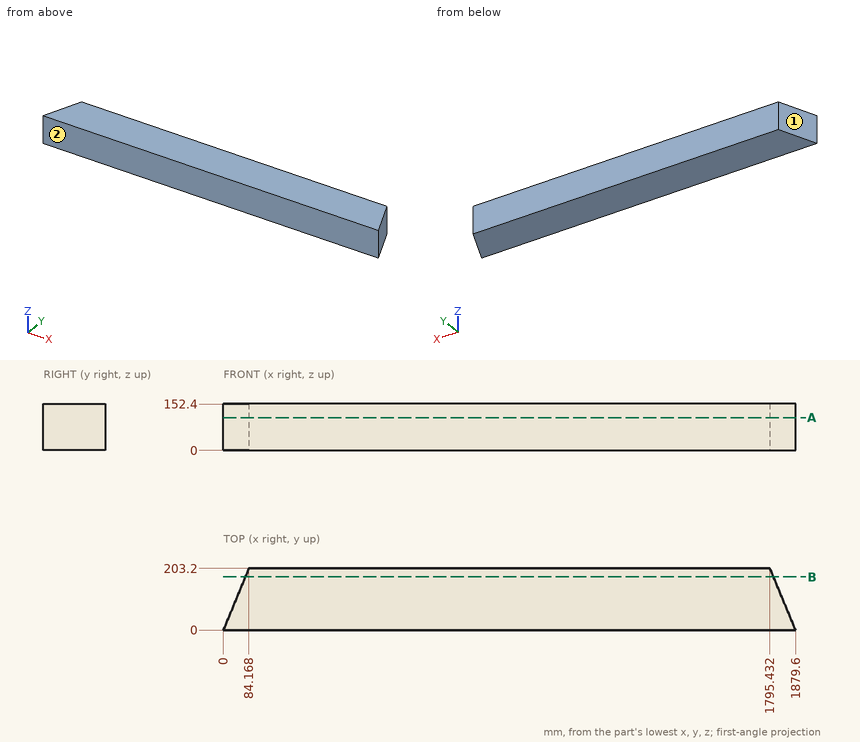
Input: dimensioned drawing with shaded views. Units: mm. Origin: part minimum x, y, z. Coordinates: 2 decimals unless noted, no trailing zeros. Write each loop counter-clockwise with the first axis right and the second up, starting at its lowest first coordinate (ties: lowest second). Pieces come first, ordered by that corner, then holes. Notation, with made-up numbers: M -8.75,-23 L 50.25,-23 A28 ccw 50.25,14 Z; hole C -17.75,-40 d5. An arc over 180 degrees is marked long. Answer as a JSON object with one key per item and string values. Group by question number.
(1) Mould query, pull axis X, two halves, no side actions, for the marked faces 1 and 2. Classes: pulls with the +X half, pulls with the -X half, needs draft (parallel to the pull), parting line crosses it, or undercut.
(2) Section B-B on y = 175. Output: boundary loops of the cut face in (x, z), plus the area to 3 significant figures.
(3) Section A-A on z = 107.5. Output: boundary loops of the cut face in (x, y), plus the area to 3 significant figures.
(4) Contact query for flat-ended pins moving along their axis: P1, Ø2, axis at y = 33.5, z = 59, coming from the -X side; P2, Ø5, axis at y = 175.5, z = 43, coming from the +X side; P3, Ø1.5, axis at y = 97.5, z = 108.5, coming from the +X side (1 decimal). Output: stop coordinate, or through.
(5) Ray query, line 1 along X through (y, z) = (144, 23.5); line 2 along X through (y, z) = (86, 131.5). Return the intervals inside material, ascending. Write a range as [from, to].
Result set:
{
 "1": {"face 1": "pulls with the -X half", "face 2": "needs draft"},
 "2": {"outline": "M 72.49,0 L 1807.11,0 L 1807.11,152.4 L 72.49,152.4 Z", "area": "264,000 mm2"},
 "3": {"outline": "M 0,0 L 1879.6,0 L 1795.43,203.2 L 84.17,203.2 Z", "area": "365,000 mm2"},
 "4": {"P1": "stops at x = 13.46", "P2": "stops at x = 1807.94", "P3": "stops at x = 1839.5"},
 "5": {"line 1": "x = [59.65, 1819.95]", "line 2": "x = [35.62, 1843.98]"}
}
